Check sheet for the drawn part. Datum: minimum x, y, z corner. Units: mm. Coordinates: 2 decimals unless noted, no trailing zeros. Order: outer loops, then holes, each group sorted by start corner. A loop starts at its lowest first (then second) coordinate and runs counter-clockwise, first axis right, second up. Notation, with made-up numbers: (-7, 14.25) -> (0, 14.25) arc R15 ccw to (0, 26.25) -> close; hole circle Ø5 at (79.25, 38.25). An arc over 180 degrees is marked (long way). Write item = value, one per line. Start each with the question number.
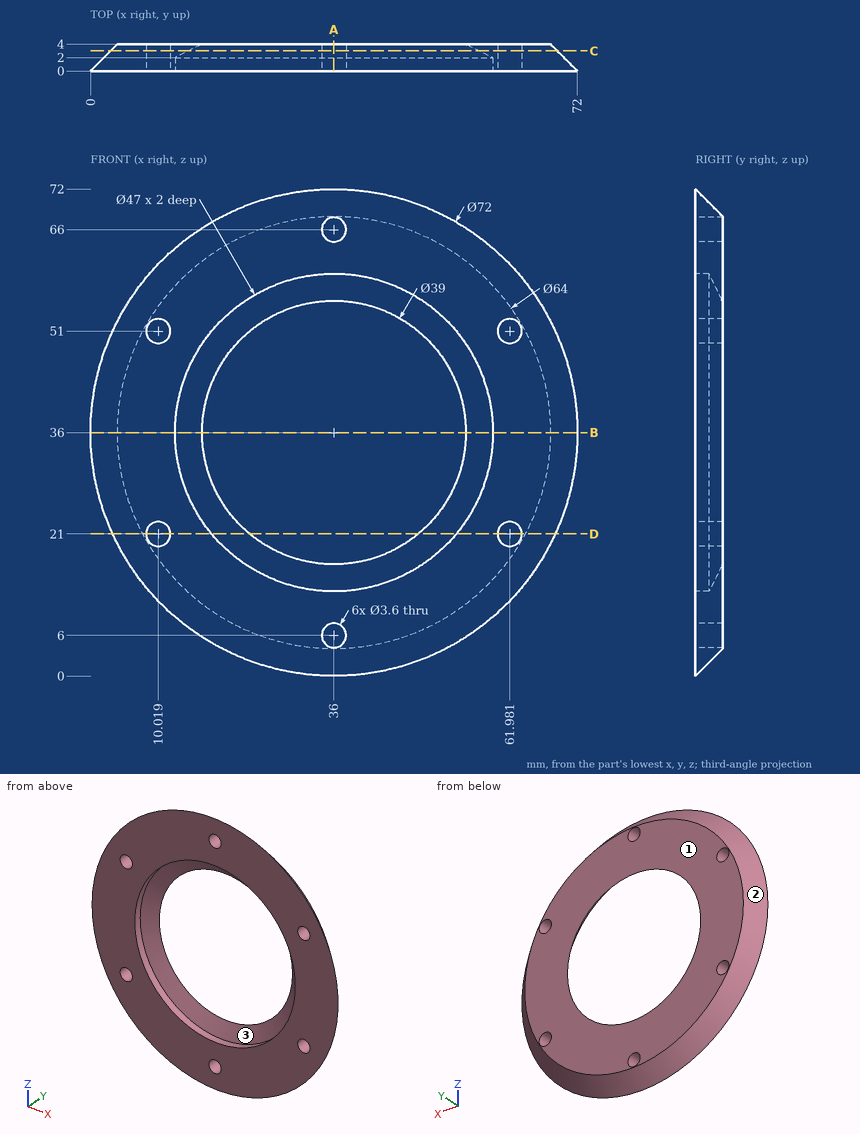
Item 1: Thickness scan on line 1 (X direction, y = 1.85, z = 51); line 2 (Z direction, x = 9, y = 0.45) (1 decimal); line 3 (X direction, y = 1.2, z = 51). Record the ranges inside material, lowest first.
Item 2: Section check C-C (y = 3). Record the boundary of the cut face in (x, z).
Item 3: Section check B-B (z = 36). Record the boundary of the cut face in (x, y).
Item 4: Gauge pin test, flat ends, axial feed: P1, Ø1, axis at x = 37.5, y = 1, coming from the +Z side; P2, Ø5, axis at x = 21.5, z = 38, coming from the -Y side; P3, Ø1.5, axis at x = 60, y = 3, coming from the -Z side; P4, Ø1, axis at x = 8.5, y = 2.5, coming from the -Z side. Record the tip position at first contact, or that the pin passes through.
Item 5: Section check D-D (z = 21). State how many separate pieces and enclosed holes the cut face has.
Item 6: Section check A-A (x = 36). Record the boundary of the cut face in (y, z), then the cut area to 3 significant figures.
Item 7: Mould release check, pull along Z, two halves, no side actions. Record for the marked faces 1, 2 and 3: pulls with the +Z half, pulls with the -Z half, needs draft (parallel to the pull), parting line crosses it, or undercut.
Filled sheet:
q1.line_1 = 5.32 to 8.22, 11.82 to 17.91, 54.09 to 60.18, 63.78 to 66.68
q1.line_2 = 12.9 to 19.5, 22.5 to 49.5, 52.5 to 59.1
q1.line_3 = 4.6 to 8.22, 11.82 to 17.91, 54.09 to 60.18, 63.78 to 67.4
q2.outline = circle Ø66 at (36, 36); hole circle Ø3.6 at (10.02, 21); hole circle Ø3.6 at (10.02, 51); hole circle Ø43 at (36, 36); hole circle Ø3.6 at (36, 6); hole circle Ø3.6 at (36, 66); hole circle Ø3.6 at (61.98, 21); hole circle Ø3.6 at (61.98, 51)
q3.outline = (0, 0) -> (12.5, 0) -> (12.5, 2) -> (16.5, 4) -> (4, 4) -> close; (55.5, 4) -> (59.5, 2) -> (59.5, 0) -> (72, 0) -> (68, 4) -> close
q4.P1 = 71.47
q4.P2 = through
q4.P3 = 12.03
q4.P4 = 15.77
q5.separate_pieces = 4
q5.enclosed_holes = 0
q6.outline = (0, 0) -> (4, 4) -> (4, 4.2) -> (0, 4.2) -> close; (0, 7.8) -> (4, 7.8) -> (4, 16.5) -> (2, 12.5) -> (0, 12.5) -> close; (0, 59.5) -> (2, 59.5) -> (4, 55.5) -> (4, 64.2) -> (0, 64.2) -> close; (0, 67.8) -> (4, 67.8) -> (4, 68) -> (0, 72) -> close
q6.area = 63.2 mm^2
q7.face_1 = needs draft
q7.face_2 = parting line crosses it
q7.face_3 = undercut
